Geometry check sheet. Reference: the model listing, model coordinates, mm. Round coordinates to 2 decimals unless told otherwise and drop trailing zeros. Write each loop counter-clockwise with the first axis right and the second up, starting at its lowest first coordinate (ties: lowest second). Pieces come first, ordered by that corner, then holes. Notation, with made-up numbers: (45, 2) -> (104, 2) arc R9 ccw to (104, 10) -> close; hole circle Ø7 at (-31, 0.25). An arc over 180 degrees is marked (long way). Return JSON: item names as keys, results as strings. Group by question number.
from build123d import *

# Parameters (mm, degrees)
SKETCH2_W               = 80
SKETCH2_H               = 12
BOSS_EXTRUDE1_DEPTH     = 13
SKETCH3_R               = 2
SKETCH3_R_2             = 1.5
CUT_EXTRUDE1_DEPTH      = 13
SKETCH4_R               = 5
CUT_EXTRUDE2_DEPTH      = 6.5
CUT_EXTRUDE2_DEPTH_BACK = 6.5


with BuildPart() as part:
    # Sketch2 → Boss-Extrude1 (new body)
    with BuildSketch(Plane(origin=(0, 0, 0), x_dir=(1, 0, 0), z_dir=(0, 1, 0))):
        Rectangle(SKETCH2_W, SKETCH2_H)
    extrude(amount=BOSS_EXTRUDE1_DEPTH)

    # Sketch3 → Cut-Extrude1 (cut)
    with BuildSketch(Plane(origin=(0, 0, 0), x_dir=(1, 0, 0), z_dir=(0, 1, 0))):
        with Locations((-36, 0)):
            Circle(SKETCH3_R)
        with Locations((-22, 0)):
            Circle(SKETCH3_R)
        with Locations((33.631617814, 0)):
            Circle(SKETCH3_R_2)
        with Locations((19.631617814, 0)):
            Circle(SKETCH3_R_2)
    extrude(amount=CUT_EXTRUDE1_DEPTH, mode=Mode.SUBTRACT)

    # Sketch4 → Cut-Extrude2 (cut, two sides)
    with BuildSketch(Plane.XY) as cut_extrude2_sk:
        with Locations((-4, 6.5)):
            Circle(SKETCH4_R)
        with Locations((5.193549115, 6.5)):
            Circle(SKETCH4_R)
    extrude(amount=CUT_EXTRUDE2_DEPTH, mode=Mode.SUBTRACT)
    extrude(cut_extrude2_sk.sketch, amount=-CUT_EXTRUDE2_DEPTH_BACK, mode=Mode.SUBTRACT)


solid = part.part
1) Sectioned sample at C-C on z = 0. Enter the section's corners in (x, y).
2) Sectioned sample at B-B on x = -22. Enter the section's corners in (y, z).
3) Mould release check, pull along X, two halves, no side actions. Record for faces 1 (the face through (10.19, 6.31, -0.08)), 2 (the face through (-1, 13, 0)), 3 (the face through (-40, 6, 0)): +X half, -X half, draft (parallel to the pull), parting line (faces both ways), or undercut.
4) Material ranges on probe 1 along X at (y, z) = (10.5, 5.75); probe 2 along X at (y, z) = (6.5, -0.5); probe 3 along X at (y, z) = (8.25, 0), recorded low to high. Write a range as [from, to].
5) Sectioned sample at D-D on y = 10.75. Enter the section's corners in (x, z), and give its area (3 significant figures).
6) Sectioned sample at A-A on y = 6.5. Enter the section's corners in (x, z), and give its area (3 significant figures).
Evaluation:
{
 "1": {"outline": "(-40, 0) -> (-38, 0) -> (-38, 13) -> (-40, 13) -> close; (-34, 0) -> (-24, 0) -> (-24, 13) -> (-34, 13) -> close; (-20, 0) -> (18.13, 0) -> (18.13, 13) -> (-20, 13) -> close; (21.13, 0) -> (32.13, 0) -> (32.13, 13) -> (21.13, 13) -> close; (35.13, 0) -> (40, 0) -> (40, 13) -> (35.13, 13) -> close; hole (0.6, 4.53) arc R5 ccw (long way) to (0.6, 8.47) arc R5 ccw (long way) to start"},
 "2": {"outline": "(0, -6) -> (13, -6) -> (13, -2) -> (0, -2) -> close; (0, 2) -> (13, 2) -> (13, 6) -> (0, 6) -> close"},
 "3": {"face 1": "undercut", "face 2": "draft", "face 3": "-X half"},
 "4": {"probe 1": "x = [-40, -7], [-1, 2.19], [8.19, 40]", "probe 2": "x = [-40, -37.94], [-34.06, -23.94], [-20.06, -9], [10.19, 18.22], [21.05, 32.22], [35.05, 40]", "probe 3": "x = [-40, -38], [-34, -24], [-20, -8.68], [9.88, 18.13], [21.13, 32.13], [35.13, 40]"},
 "5": {"outline": "(-40, -6) -> (-6.63, -6) -> (-6.63, 6) -> (-40, 6) -> close; (-1.37, -6) -> (2.56, -6) -> (2.56, 6) -> (-1.37, 6) -> close; (7.83, -6) -> (40, -6) -> (40, 6) -> (7.83, 6) -> close; hole circle Ø4 at (-36, 0); hole circle Ø4 at (-22, 0); hole circle Ø3 at (19.63, 0); hole circle Ø3 at (33.63, 0)", "area": "794 mm2"},
 "6": {"outline": "(-40, -6) -> (-9, -6) -> (-9, 6) -> (-40, 6) -> close; (10.19, -6) -> (40, -6) -> (40, 6) -> (10.19, 6) -> close; hole circle Ø4 at (-36, 0); hole circle Ø4 at (-22, 0); hole circle Ø3 at (19.63, 0); hole circle Ø3 at (33.63, 0)", "area": "690 mm2"}
}
